Check sheet for the modelled part. Datum: model origin and axes. Units: mm. A direction names the side the tool comes from. Give positions to 0.01 mm unless a question says otherwise; leave off trailing zeros. Write each loop counter-clockwise with the first axis right and the second up, starting at its lowest first coordinate (ties: lowest second). Pieces come first, ordered by that corner, then holes. Notation, with made-up numbers: M 21,22 L 50,22 A20 ccw 50,61 Z; hole C -15.75,45.5 d4. An arc over 180 degrees is marked long. One line per item, written item: value. Start each with the question number.
from build123d import *

# Parameters (mm, degrees)
SKETCH_W  = 40
SKETCH_H  = 40
SKETCH_R  = 2.25
PAD_DEPTH = 5


with BuildPart() as part:
    # Sketch → Pad (new body)
    with BuildSketch(Plane.XY):
        Rectangle(SKETCH_W, SKETCH_H)
        with Locations((0, 13.75)):
            Circle(SKETCH_R, mode=Mode.SUBTRACT)
        with Locations((0, -13.75)):
            Circle(SKETCH_R, mode=Mode.SUBTRACT)
        with BuildLine():
            ThreePointArc((-4.999983, 4.5), (-9.499983, 9e-06), (-5, -4.5))
            Line((-5, -4.5), (5, -4.5))
            ThreePointArc((5, -4.5), (9.499983, 9e-06), (4.999983, 4.5))
            Line((-4.999983, 4.5), (4.999983, 4.5))
        make_face(mode=Mode.SUBTRACT)
    extrude(amount=PAD_DEPTH)


solid = part.part
1) Cross-section at A-A (x = 0). Record the boundary of the cut face in (y, z).
2) Cross-section at B-B (y = 0). Record the boundary of the cut face in (x, z).
3) Cross-section at D-D (y = 13.75). Record the boundary of the cut face in (x, z), plus the area to 4 significant figures.
4) Material ranges on L1, parallel to Y at x = 0, z = 1.15; L2, parallel to Y at x = -0.5, z = 1.2; L3, parallel to Y at x = 7, z = 0.5, recorded low to high. Write a range as from..to.
5) Draft check along X on faces 1 (the flat face through (0, 5, 0)), 2 (the flat face through (0, 4.5, 2)), 3 (the flat face through (-20, 0, 2)), 4 (the flat face through (20, 0, 2)). Enter one of: released by +X, released by -X, zero draft, split by the parting line, or undercut.
6) Tool access check on faces 5 (the cylindrical face through (9.5, -0.1, 2.5)), 6 (the flat face through (0, 20, 2)). Record the directions out of +Z, -Z, +X, -X, +Y, -Y that give a thin tool (end or side, any length) a straight path to the whole face; none if there is none.
7) Cross-section at C-C (z = 3.7). Record the boundary of the cut face in (x, y), plus the area to 3 significant figures.
Data:
1. outline: M -20,0 L -16,0 L -16,5 L -20,5 Z; M -11.5,0 L -4.5,0 L -4.5,5 L -11.5,5 Z; M 4.5,0 L 11.5,0 L 11.5,5 L 4.5,5 Z; M 16,0 L 20,0 L 20,5 L 16,5 Z
2. outline: M -20,0 L -9.5,0 L -9.5,5 L -20,5 Z; M 9.5,0 L 20,0 L 20,5 L 9.5,5 Z
3. outline: M -20,0 L -2.25,0 L -2.25,5 L -20,5 Z; M 2.25,0 L 20,0 L 20,5 L 2.25,5 Z
3. area: 177.5 mm2
4. L1: y = -20..-16, -11.5..-4.5, 4.5..11.5, 16..20
4. L2: y = -20..-15.94, -11.56..-4.5, 4.5..11.56, 15.94..20
4. L3: y = -20..-4.03, 4.03..20
5. face 1: zero draft
5. face 2: undercut
5. face 3: released by -X
5. face 4: released by +X
6. face 5: +Z, -Z
6. face 6: +Z, -Z, +X, -X, +Y
7. outline: M -20,-20 L 20,-20 L 20,20 L -20,20 Z; hole M -5,-4.5 L 5,-4.5 A4.5 ccw 5,4.5 L -5,4.5 A4.5 ccw Z; hole C 0,-13.75 d4.5; hole C 0,13.75 d4.5
7. area: 1,410 mm2
